Answer from the drawing. Dimensions are ordinates in mm from the lowest x, y and z of the part. Give positions to 0.01 mm unless a question says otherwise; leave off trailing zeros. Order: outer loops, then holes, each group sorted by start corner. A loop starts at its lowest first (then second) coordinate and runs counter-clockwise, first axis right, second up.
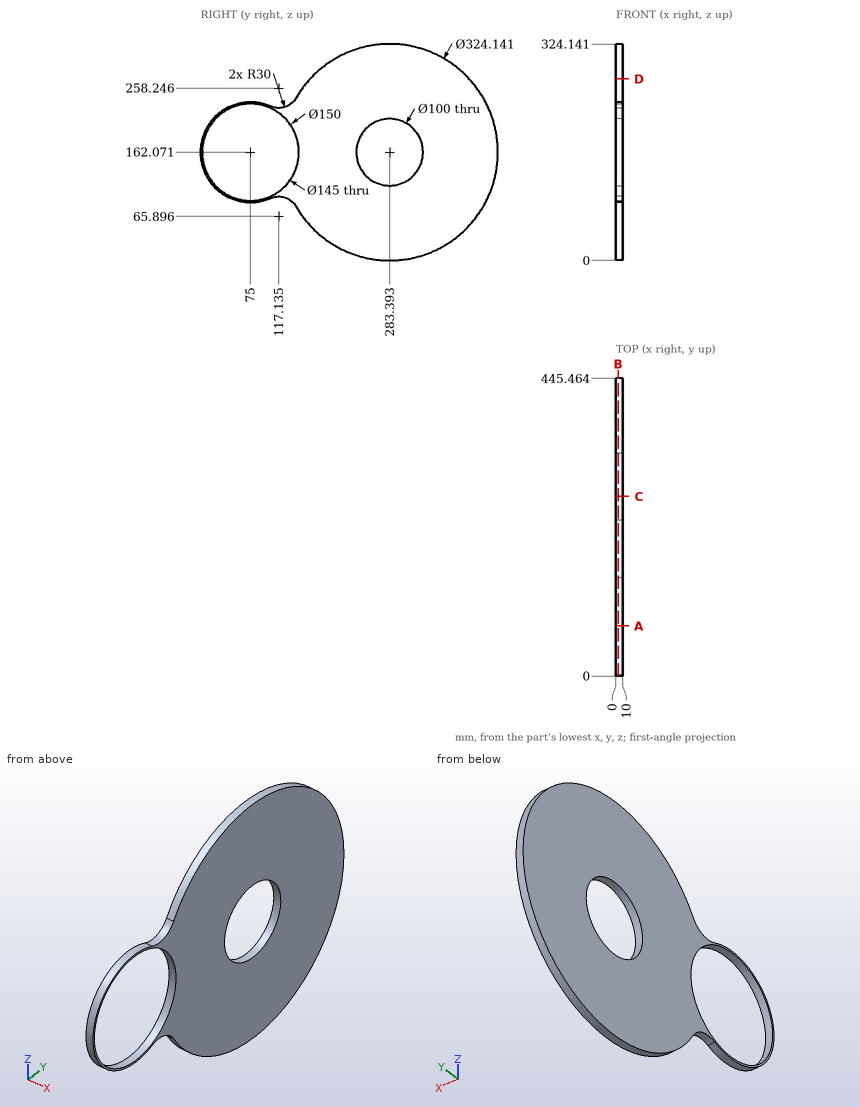
1) The part is cut by section B-B on x = 3.25. Determine the outline of the cut face in (y, z) (1 decimal), and give its area (3 significant figures).
Final values:
outline: (105.1, 93.4) arc R30 cw to (143.1, 80.9) arc R162.1 ccw (long way) to (143.1, 243.2) arc R30 cw to (105.1, 230.8) arc R75 ccw (long way) to start; hole circle Ø145 at (75, 162.1); hole circle Ø100 at (283.4, 162.1)
area: 74,300 mm2
2) Consider L1, parallel to Y at x = 4.75, z = 191 (1 decimal); L2, parallel to Y at x = 6.5, z = 178; L3, parallel to Z at x = 4, y = 239.5 (1 decimal). Determine where each line is inside the solid, lowest interval first.
Final values:
L1: y = 5.8 to 8.5, 141.5 to 242.6, 324.2 to 442.9
L2: y = 1.71 to 4.27, 145.73 to 236, 330.79 to 444.68
L3: z = 6.1 to 138.1, 186 to 318.1
3) The part is cut by section D-D on z = 272. Determine the outline of the cut face in (x, y), and give its area (3 significant figures).
Final values:
outline: (0, 164.3) - (10, 164.3) - (10, 402.48) - (0, 402.48) - close
area: 2,380 mm2
4) The part is cut by section C-C on y = 269. Determine the outline of the cut face in (x, z) (1 decimal).
Final values:
outline: (0, 0.6) - (10, 0.6) - (10, 114.2) - (0, 114.2) - close; (0, 210) - (10, 210) - (10, 323.5) - (0, 323.5) - close
5) Given pin 1 (6 mm diameter, centred on x = 5, y = 327, fed in from +Z); pin 2 (5 mm diameter, centred on x = 6.5, y = 66, fed in from -Z); pin 3 (1 mm diameter, centred on x = 9, y = 384.5, fed in from -Z), each flat-ended and moving along its own axis, determine where each tip first touches the part or whether it passes through.
Final values:
pin 1: stops at z = 318.97
pin 2: stops at z = 87.35
pin 3: stops at z = 35.01
6) The part is cut by section A-A on y = 75. Determine the outline of the cut face in (x, z).
Final values:
outline: (0, 87.07) - (10, 87.07) - (10, 89.57) - (0, 89.57) - close; (0, 234.57) - (10, 234.57) - (10, 237.07) - (0, 237.07) - close
